from build123d import *

# Parameters (mm, degrees)
F0_R      = 30
F1_DEPTH  = 5
F2_R      = 5
F3_DEPTH  = 10
F4_R      = 1.85
F5_DEPTH  = 15
F6_R      = 3
F6_R_2    = 1.85
F7_DEPTH  = 1.5
F9_DEPTH  = 5
F10_R     = 33
F10_R_2   = 30
F10_R_3   = 1.85
F11_DEPTH = 0.7


with BuildPart() as f1:
    # F0 (on Top) → F1 (new body)
    with BuildSketch(Plane.XY):
        Circle(F0_R)
    extrude(amount=F1_DEPTH)

    # F2 (on face) → F3 (join)
    with BuildSketch(Plane.XY.offset(5)):
        Circle(F2_R)
    extrude(amount=F3_DEPTH)

    # F4 (on face) → F5 (cut, through all)
    with BuildSketch(Plane.XY.offset(15)):
        Circle(F4_R)
    extrude(amount=-F5_DEPTH, mode=Mode.SUBTRACT)

    # F6 (on face) → F7 (join)
    with BuildSketch(Plane.XY.offset(15)):
        Circle(F6_R)
        Circle(F6_R_2, mode=Mode.SUBTRACT)
    extrude(amount=F7_DEPTH)

    # F8 (on face) → F9 (cut, through all)
    with BuildSketch(Plane.XY.offset(5)):
        with BuildLine():
            Line((6.3245553203, 1.5), (28.9611809151, 1.5))
            ThreePointArc((28.9611809151, 1.5), (20.5060966544, 20.5060966544), (1.5, 28.9611809151))
            Line((1.5, 28.9611809151), (1.5, 6.3245553203))
            ThreePointArc((1.5, 6.3245553203), (4.5961940777, 4.5961940777), (6.3245553203, 1.5))
        make_face()
        with BuildLine():
            Line((-1.5, 6.3245553203), (-1.5, 28.9611809151))
            ThreePointArc((-1.5, 28.9611809151), (-20.5060966544, 20.5060966544), (-28.9611809151, 1.5))
            Line((-28.9611809151, 1.5), (-6.3245553203, 1.5))
            ThreePointArc((-6.3245553203, 1.5), (-4.5961940777, 4.5961940777), (-1.5, 6.3245553203))
        make_face()
        with BuildLine():
            ThreePointArc((-28.9611809151, -1.5), (-20.5060966544, -20.5060966544), (-1.5, -28.9611809151))
            Line((-1.5, -28.9611809151), (-1.5, -6.3245553203))
            ThreePointArc((-1.5, -6.3245553203), (-4.5961940777, -4.5961940777), (-6.3245553203, -1.5))
            Line((-6.3245553203, -1.5), (-28.9611809151, -1.5))
        make_face()
        with BuildLine():
            ThreePointArc((1.5, -28.9611809151), (20.5060966544, -20.5060966544), (28.9611809151, -1.5))
            Line((28.9611809151, -1.5), (6.3245553203, -1.5))
            ThreePointArc((6.3245553203, -1.5), (4.5961940777, -4.5961940777), (1.5, -6.3245553203))
            Line((1.5, -6.3245553203), (1.5, -28.9611809151))
        make_face()
    extrude(amount=-F9_DEPTH, mode=Mode.SUBTRACT)

    # F10 (on face) → F11 (join)
    with BuildSketch(Plane(origin=(0, 0, 0), x_dir=(1, 0, 0), z_dir=(0, 0, -1))):
        Circle(F10_R)
        Circle(F10_R_2, mode=Mode.SUBTRACT)
        Circle(F10_R_2)
        with BuildLine():
            Line((-1.5, -6.3245553203), (-1.5, -28.9611809151))
            ThreePointArc((-1.5, -28.9611809151), (-20.5060966544, -20.5060966544), (-28.9611809151, -1.5))
            Line((-28.9611809151, -1.5), (-6.3245553203, -1.5))
            ThreePointArc((-6.3245553203, -1.5), (-4.5961940777, -4.5961940777), (-1.5, -6.3245553203))
        make_face(mode=Mode.SUBTRACT)
        with BuildLine():
            ThreePointArc((28.9611809151, -1.5), (20.5060966544, -20.5060966544), (1.5, -28.9611809151))
            Line((1.5, -28.9611809151), (1.5, -6.3245553203))
            ThreePointArc((1.5, -6.3245553203), (4.5961940777, -4.5961940777), (6.3245553203, -1.5))
            Line((6.3245553203, -1.5), (28.9611809151, -1.5))
        make_face(mode=Mode.SUBTRACT)
        with BuildLine():
            ThreePointArc((-1.5, 6.3245553203), (-4.5961940777, 4.5961940777), (-6.3245553203, 1.5))
            Line((-6.3245553203, 1.5), (-28.9611809151, 1.5))
            ThreePointArc((-28.9611809151, 1.5), (-20.5060966544, 20.5060966544), (-1.5, 28.9611809151))
            Line((-1.5, 28.9611809151), (-1.5, 6.3245553203))
        make_face(mode=Mode.SUBTRACT)
        Circle(F10_R_3, mode=Mode.SUBTRACT)
        with BuildLine():
            Line((1.5, 6.3245553203), (1.5, 28.9611809151))
            ThreePointArc((1.5, 28.9611809151), (20.5060966544, 20.5060966544), (28.9611809151, 1.5))
            Line((28.9611809151, 1.5), (6.3245553203, 1.5))
            ThreePointArc((6.3245553203, 1.5), (4.5961940777, 4.5961940777), (1.5, 6.3245553203))
        make_face(mode=Mode.SUBTRACT)
    extrude(amount=F11_DEPTH)


solid = f1.part
Can you work these out from the model? Positions are in its coordinate system, mm. A direction names the side the tool comes from. Coordinates: 2 decimals unless noted, no trailing zeros. Order: outer loops, then holes, each group sorted by start corner. A loop starts at its lowest first (then second) coordinate and runs counter-clockwise, first axis right, second up. Notation, with made-up numbers: (-3, -19.75) - (29, -19.75) arc R7 ccw to (29, -11.75) - close; hole circle Ø2 at (-9.75, -31.5). An arc over 180 degrees is marked (long way). Answer as a JSON object with one key per item and string values. Group by question number.
Q1. Imagine slicing it at D-D (y = -18.5). Please give me the cut outline in (x, z).
Q2. We'd pull the mould along X, two halves only. Please class faces 4 (the face through (17, 1.5, 2)), 5 (the face through (-0.1, -3.3, 15)), 6 (the face through (30.5, 12.6, -0.3)): +X half, -X half, draft (parallel to the pull), parting line (faces both ways), or undercut.
Q3. On a 3-axis mill with a long thin cutter (end or side, diameter ignored), from which of +Z, -Z, +X, -X, +Y, -Y can I reach the whole of each face in a straight line? I mean faces 1 (the face through (0, 7, -0.7)), 2 (the face through (-1.5, 17, 2)), 3 (the face through (-1.08, -4.88, 9.93)). Say none if no direction works.
Q4. I need wall thicknesses on line 1 (Y direction, x = 0, z = 6.25); line 2 (Y direction, x = -14, z = 1.25); line 3 (Y direction, x = 5, z = 4). Which ranges of each line are inside material? Lowest first, please. Write a range as from..to.
Q5. Imagine slicing it at B-B (x = 25.5). Please give me the cut outline in (y, z), and give its area (3 significant figures).
Q6. Will these pins go through, and if not, where does the flat tip stop? P1, Ø4.5, axis at x = 23, z = 1, coming from the -Y side; P2, Ø4.5, axis at x = 23, z = 2.5, coming from the +Y side; P3, Ø1.7, axis at x = -18.5, z = 2, coming from the -Y side.
Q7. Imagine slicing it at A-A (y = 0). Please give me the cut outline in (x, z).
Determined:
{
 "1": {"outline": "(-27.33, -0.7) - (-22.33, -0.7) - (-22.33, 5) - (-23.62, 5) - (-23.62, 0) - (-27.33, 0) - close; (-1.5, -0.7) - (1.5, -0.7) - (1.5, 5) - (-1.5, 5) - close; (22.33, -0.7) - (27.33, -0.7) - (27.33, 0) - (23.62, 0) - (23.62, 5) - (22.33, 5) - close"},
 "2": {"face 4": "undercut", "face 5": "draft", "face 6": "parting line"},
 "3": {"face 1": "-Z, +X, -X, +Y, -Y", "face 2": "+Z, -Z", "face 3": "+Z"},
 "4": {"line 1": "y = -5..-1.85, 1.85..5", "line 2": "y = -26.53..-25.4, -1.5..1.5, 25.4..26.53", "line 3": "y = -29.58..-28.57, -4.15..4.15, 28.57..29.58"},
 "5": {"outline": "(-20.95, -0.7) - (-13.81, -0.7) - (-13.81, 5) - (-15.8, 5) - (-15.8, 0) - (-20.95, 0) - close; (-1.5, -0.7) - (1.5, -0.7) - (1.5, 5) - (-1.5, 5) - close; (13.81, -0.7) - (20.95, -0.7) - (20.95, 0) - (15.8, 0) - (15.8, 5) - (13.81, 5) - close", "area": "47.0 mm2"},
 "6": {"P1": "stops at y = -25.47", "P2": "stops at y = 21.67", "P3": "stops at y = -24.26"},
 "7": {"outline": "(-33, -0.7) - (-1.85, -0.7) - (-1.85, 16.5) - (-3, 16.5) - (-3, 15) - (-5, 15) - (-5, 5) - (-30, 5) - (-30, 0) - (-33, 0) - close; (1.85, -0.7) - (33, -0.7) - (33, 0) - (30, 0) - (30, 5) - (5, 5) - (5, 15) - (3, 15) - (3, 16.5) - (1.85, 16.5) - close"}
}
